Geometry: final body of the model. Coordinates: model frame, mm. Face numbers are marked on the shaded views. Coordinates: 2 decimals unless noted, no trailing zeros. Order: outer loops, then holes, each group sorted by start corner. A loop starts at its lowest first (then second) coordinate and runs counter-clockwise, first axis right, second up. Notation, with made-up numbers: M 77,-24 L 121,-24 A21 cw 121,3 Z; hole C 29,-21.5 d3. An arc over 180 degrees is marked long. Write item = value, one per line.
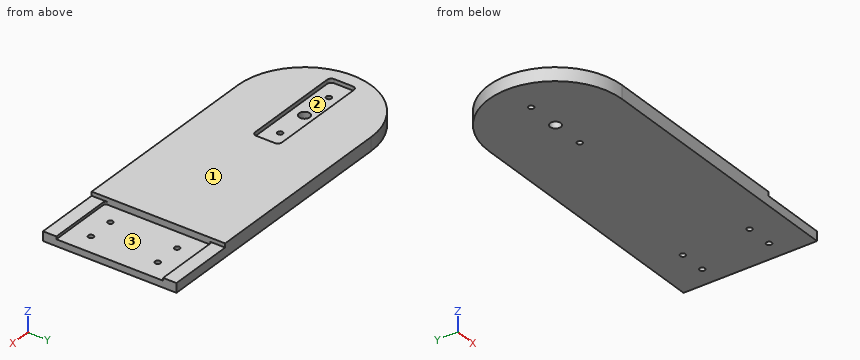
Autodesk Inventor part; units mm, degrees
ref_plane "YZ Plane" through (0, 0, 0) normal (1, 0, 0) x (0, 1, 0)
ref_plane "XZ Plane" through (0, 0, 0) normal (0, 1, 0) x (-1, 0, 0)
ref_plane "XY Plane" through (0, 0, 0) normal (0, 0, 1) x (1, 0, 0)
sketch "Sketch1" plane through (0, 0, 0) normal (0, 0, 1) x (1, 0, 0)
  line L0 (232.6946, -90.5389) -> (32.6946, -90.5389)
  line L1 (-17.3054, -40.5389) -> (-17.3054, -40.5389)
  line L2 (32.6946, 9.4611) -> (232.6946, 9.4611)
  line L3 (232.6946, 9.4611) -> (232.6946, -90.5389)
  circle A0 centre (32.6946, -40.5389) radius 4
  arc A1 (-17.3054, -40.5389) -> (32.6946, -90.5389) centre (32.6946, -40.5389) ccw
  arc A2 (32.6946, 9.4611) -> (-17.3054, -40.5389) centre (32.6946, -40.5389) ccw
  point P0 (0, 0)
  point P1 (-17.3054, 9.4611)
  point P2 (-17.3054, -90.5389)
  dimension "d0" = 250
  dimension "d1" = 100
  dimension "d2" = 8
  dimension "d3" = 50
  dimension "d4" = 50
  dimension "d5" = 50
extrude "Extrusion1" add sketch "Sketch1" along normal blind 10
sketch "Sketch2" plane through (0, 0, 10) normal (0, 0, 1) x (1, 0, 0)
  line L0 (32.6946, 9.4611) -> (232.6946, 9.4611)
  line L1 (232.6946, -90.5389) -> (182.6946, -90.5389)
  line L2 (182.6946, -90.5389) -> (182.6946, 9.4611)
  line L3 (182.6946, 9.4611) -> (232.6946, 9.4611)
  line L4 (232.6946, 9.4611) -> (232.6946, -90.5389)
  point P0 (0, 0)
  dimension "d8" = 50
extrude "Extrusion2" cut sketch "Sketch2" against normal blind 5
sketch "Sketch3" plane through (0, 0, 5) normal (0, 0, 1) x (1, 0, 0)
  line L0 (182.6946, 9.4611) -> (232.6946, 9.4611)
  line L1 (182.6946, 9.4611) -> (182.6946, -90.5389)
  line L2 (232.6946, -90.5389) -> (182.6946, -90.5389)
  line L3 (232.6946, 9.4611) -> (232.6946, -90.5389)
  point P0 (0, 0)
  point P1 (197.6946, -65.5389)
  point P2 (197.6946, -15.5389)
  point P3 (217.6946, -15.5389)
  point P4 (217.6946, -65.5389)
  dimension "d11" = 15
  dimension "d12" = 25
  dimension "d13" = 25
  dimension "d14" = 15
hole "Hole1" at (197.6946, -65.5389, 5) at (197.6946, -15.5389, 5) at (217.6946, -15.5389, 5) at (217.6946, -65.5389, 5) direction (0, 0, -1) diameter 4 end through all
sketch "Sketch4" plane through (0, 0, 10) normal (0, 0, 1) x (1, 0, 0)
  arc A0 (32.6946, 9.4611) -> (32.6946, -90.5389) centre (32.6946, -40.5389) ccw
  point P0 (0, 0)
  point P1 (7.6946, -40.5389)
  point P2 (57.6946, -40.5389)
  dimension "d22" = 25
  dimension "d23" = 25
hole "Hole2" at (7.6946, -40.5389, 10) at (57.6946, -40.5389, 10) direction (0, 0, -1) diameter 4 end through all
sketch "Sketch5" plane through (0, 0, 10) normal (0, 0, 1) x (1, 0, 0)
  circle A0 centre (57.6946, -40.5389) radius 2
  circle A1 centre (7.6946, -40.5389) radius 2
  arc A2 (32.6946, 9.4611) -> (32.6946, -90.5389) centre (32.6946, -40.5389) ccw
  circle A3 centre (32.6946, -40.5389) radius 4
  line L0 (72.6946, -50.5389) -> (-7.3054, -50.5389)
  line L1 (-7.3054, -50.5389) -> (-7.3054, -30.5389)
  line L2 (-7.3054, -30.5389) -> (72.6946, -30.5389)
  line L3 (72.6946, -30.5389) -> (72.6946, -50.5389)
  point P0 (0, 0)
  dimension "d35" = 80
  dimension "d36" = 20
  dimension "d37" = 40
  dimension "d38" = 10
extrude "Extrusion3" cut sketch "Sketch5" against normal blind 3
sketch "Sketch6" plane through (0, 0, 5) normal (0, 0, 1) x (1, 0, 0)
  line L0 (232.6946, 9.4611) -> (232.6946, -90.5389)
  line L1 (182.6946, -90.5389) -> (232.6946, -90.5389)
  line L2 (232.6946, -90.5389) -> (232.6946, -80.5389)
  line L3 (232.6946, -80.5389) -> (182.6946, -80.5389)
  line L4 (182.6946, -80.5389) -> (182.6946, -90.5389)
  line L5 (182.6946, 9.4611) -> (232.6946, 9.4611)
  line L6 (232.6946, 9.4611) -> (232.6946, -0.5389)
  line L7 (232.6946, -0.5389) -> (182.6946, -0.5389)
  line L8 (182.6946, -0.5389) -> (182.6946, 9.4611)
  point P0 (0, 0)
  dimension "d41" = 10
  dimension "d42" = 10
extrude "Extrusion4" add sketch "Sketch6" along normal blind 2
fillet "Fillet1" radius 2 2 edges at (182.6946, -0.5389, 6) (182.6946, -80.5389, 6)
fillet "Fillet2" radius 3 4 edges at (-7.3054, -30.5389, 8.5) (-7.3054, -50.5389, 8.5) (72.6946, -30.5389, 8.5) (72.6946, -50.5389, 8.5)
equation "\"d4\" = 0.5 * d1"
equation "\"d37\" = 0.5 * d35"
equation "\"d38\" = 0.5 * d36"
properties part number "plancha base"
1) Pin query (flat end, axial travel): pin 1 (4.5 mm diameter, centred on x = 7.69, y = -40.54, fed in from +Z); pin 2 (2 mm diameter, centred on y = -33.5, z = 9, fed in from +X); pin 3 (3.5 mm diameter, centred on x = 57.69, y = -40.54, fed in from -Z); pin 4 (0.9 mm diameter, centred on x = 16.5, z = 8, fed in from -Y). Return the tip coordinate at first contact, or that it passes through.
Numbers:
pin_1 = 7
pin_2 = 182.69
pin_3 = through
pin_4 = -88
2) Section B-B, the plane z = 2. Return loops of the section in (x, y), and give its area (3 significant figures).
Numbers:
outline = M 32.69,-90.54 L 232.69,-90.54 L 232.69,9.46 L 32.69,9.46 A50 ccw Z; hole C 7.69,-40.54 d4; hole C 32.69,-40.54 d8; hole C 57.69,-40.54 d4; hole C 197.69,-65.54 d4; hole C 197.69,-15.54 d4; hole C 217.69,-65.54 d4; hole C 217.69,-15.54 d4
area = 23,800 mm²
3) Mould query, pull axis Y, two halves, no side actions, for the marked faces 1, 2 and 3. Classes: pulls with the +Y half, pulls with the -Y half, needs draft (parallel to the pull), parting line crosses it, or undercut.
Numbers:
face_1 = needs draft
face_2 = undercut
face_3 = undercut
4) Section C-C, the plane y = -54.5. Return loops of the section in (x, z).
Numbers:
outline = M -15.32,0 L 232.69,0 L 232.69,5 L 182.69,5 L 182.69,10 L -15.32,10 Z
5) Section A-A, the plane x = 63.5. Return loops of the section in (y, z).
Numbers:
outline = M -90.54,0 L 9.46,0 L 9.46,10 L -30.54,10 L -30.54,7 L -50.54,7 L -50.54,10 L -90.54,10 Z
6) Section D-D, the plane x = -1. Return loops of the section in (y, z), and give its area (3 significant figures).
Numbers:
outline = M -77.48,0 L -3.6,0 L -3.6,10 L -30.54,10 L -30.54,7 L -50.54,7 L -50.54,10 L -77.48,10 Z
area = 679 mm²
7) Line query: L1, parallel to Y at x = 32.5, z = 6.5; L2, parallel to Y at x = 217.5, z = 6.75; L3, parallel to X at y = -38.5, z = 1.5. Output: solid intervals per line, ascending.
Numbers:
L1 = -90.54 to -44.53, -36.54 to 9.46
L2 = -90.54 to -80.54, -0.54 to 9.46
L3 = -17.26 to 29.25, 36.14 to 232.69
